For this review, take the finished solid that the model builds, in its own axes (mm). A direction names the side the tool comes from. Give positions to 0.01 mm unless a question says otherwise; leave off trailing zeros. Write each loop counter-clockwise with the first axis right and the second up, starting at its lowest first coordinate (ties: lowest second). Pieces come first, ordered by that corner, then holes. Notation, with made-up numbers: M -6.5,48 L 40.5,48 A22 cw 40.5,60 Z; hole C 50.25,5 d8. An arc over 180 degrees is marked long. One line per item, written item: value. Start each with the question number.
Item 1: Consider section C-C, the plane z = 11.25. Write out the cut boundary in (x, y), and give its area (3 significant figures).
Item 2: Consider section B-B, the plane y = 25.75. Write out the cut boundary in (x, z), and give its area (3 significant figures).
Item 3: Consider section A-A, the plane x = 24.75. Write out the cut boundary in (y, z), and give its area (3 significant figures).
Item 4: Clearance check with flat-ended pins moving along their axes: pin 1 Ø1 at (x, z) = (18.5, 12.5) entering from -Y; pin 2 Ø6 at (y, z) = (24, 27) entering from +X; pin 3 Ø8 at (x, z) = (23, 22) entering from -Y. State where each tip first meets the part, or that it passes through.
Item 5: Consider section D-D, the plane x = 26.5. Write out the cut boundary in (y, z).
Item 6: Tool access review of faces 4 (the face through (25, 25, 7)), 5 (the face through (25, 25, 12)), 6 (the face through (23.405, 34.362, 14.79)): name each direction out of +Z, -Z, +X, -X, +Y, -Y from which nothing blocks a thin tool from reaching the whole face with its end or side.
Item 7: To check wall thickness, follow probe 1 along Z at (x, y) = (26.75, 23.5); probe 2 along X at (y, z) = (26, 18.5); probe 3 along Y at (x, z) = (18.25, 13.5). State the ranges of each line that lie inside material, in increasing order.
Item 8: Mouldability with a two-part tool opening along Y and no side actions: class faces 1 (the face through (15.793, 25.992, 14.79)), 2 (the face through (21, 30, 30)), 3 (the face through (26.249, 26.653, 9.535)) as released by +Y, released by -Y, zero draft, split by the parting line, or undercut.
```python
from build123d import *

# Parameters (mm, degrees)
BOSS_EXTRUDE2_DEPTH = 30
SKETCH3_W           = 8
SKETCH3_H           = 30
BOSS_EXTRUDE3_DEPTH = 10
BOSS_EXTRUDE4_DEPTH = 23
CUT_EXTRUDE1_DEPTH  = 18


with BuildPart() as part:
    # Sketch2 → Boss-Extrude2 (new body)
    with BuildSketch(Plane.XY):
        Polygon((16.826264571, 24.026772498), (14.730988717, 28.012523819), (21.495359976, 23.741308364), (16.995960151, 23.919621906), align=None)
    extrude(amount=BOSS_EXTRUDE2_DEPTH)

    # Sketch3 → Boss-Extrude3 (add)
    with BuildSketch(Plane(origin=(16.845028917, 26.677659006, 0), x_dir=(0.845546407, -0.533901932, 0), z_dir=(0.533901932, 0.845546407, 0))):
        with Locations((1.499794001, -15)):
            Rectangle(SKETCH3_W, SKETCH3_H)
    extrude(amount=BOSS_EXTRUDE3_DEPTH)

    # Sketch5 → Boss-Extrude4 (add)
    with BuildSketch(Plane.XY.offset(30)):
        Polygon((24.164869635, 27.969040401), (28.392601672, 25.299530741), (25.723092013, 21.071798704), (21.495359976, 23.741308364), align=None)
    extrude(amount=-BOSS_EXTRUDE4_DEPTH)

    # Sketch6 → Cut-Extrude1 (cut)
    with BuildSketch(Plane.XY.offset(30)):
        Polygon((21.495359976, 23.741308364), (24.164869635, 27.969040401), (28.392601672, 25.299530741), (25.723092013, 21.071798704), align=None)
    extrude(amount=-CUT_EXTRUDE1_DEPTH, mode=Mode.SUBTRACT)


solid = part.part
```
Model answer:
1. outline: M 14.73,28.01 L 16.83,24.03 L 17,23.92 L 21.5,23.74 L 25.72,21.07 L 28.39,25.3 L 24.16,27.97 L 26.83,32.2 L 20.07,36.47 Z
1. area: 114 mm2
2. outline: M 15.92,0 L 22.76,0 L 22.76,7 L 27.68,7 L 27.68,12 L 22.76,12 L 22.76,30 L 15.92,30 Z
2. area: 230 mm2
3. outline: M 21.69,7 L 27.6,7 L 27.6,12 L 21.69,12 Z; M 28.9,0 L 33.51,0 L 33.51,30 L 28.9,30 Z
3. area: 168 mm2
4. pin 1: stops at y = 23.84
4. pin 2: stops at x = 23.55
4. pin 3: stops at y = 23.74
5. outline: M 22.3,7 L 26.49,7 L 26.49,12 L 22.3,12 Z; M 31.67,0 L 32.41,0 L 32.41,30 L 31.67,30 Z
6. face 4: -Z, +X, -Y
6. face 5: +Z, +X, -Y
6. face 6: +Z, -Z, +X, +Y
7. probe 1: z = 7 to 12
7. probe 2: x = 15.79 to 22.92
7. probe 3: y = 23.87 to 33.59
8. face 1: released by -Y
8. face 2: zero draft
8. face 3: undercut
